from build123d import *

# Parameters (mm, degrees)
F0_R     = 30
F1_DEPTH = 3
F2_SIZE  = 2.99999
F3_R     = 19.125
F4_DEPTH = 3.001
F5_R     = 24.75
F5_R_2   = 22.75
F6_DEPTH = 20


# Not quite as in the source:
# - a fillet or chamfer is up to 0.001 mm smaller than in the source, because OpenCascade refuses the exact size


with BuildPart() as f1:
    # F0 (on Top) → F1 (new body)
    with BuildSketch(Plane.XY):
        Circle(F0_R)
    extrude(amount=F1_DEPTH)

    # F2 (size 3 in the source; OpenCascade refuses exactly that, so slightly less here)
    f2_edges = [f1.edges().sort_by_distance(p)[0] for p in [
        (-30, 0, 3),
    ]]
    chamfer(f2_edges, length=F2_SIZE)

    # F3 (on face) → F4 (cut, through all)
    with BuildSketch(Plane.XY.offset(3)):
        Circle(F3_R)
    extrude(amount=-F4_DEPTH, mode=Mode.SUBTRACT)

    # F5 (on face) → F6 (join)
    with BuildSketch(Plane(origin=(0, 0, 0), x_dir=(1, 0, 0), z_dir=(0, 0, -1))):
        Circle(F5_R)
        Circle(F5_R_2, mode=Mode.SUBTRACT)
    extrude(amount=F6_DEPTH)


solid = f1.part
Here's how the part is built. I have some questions about the finished solid (model axes, mm). A direction names the side the tool comes from. Give positions to 0.01 mm unless a question says otherwise; leave off trailing zeros. Write each loop counter-clockwise with the first axis right and the second up, starting at its lowest first coordinate (ties: lowest second). Pieces come first, ordered by that corner, then holes. Notation, with made-up numbers: (20.5, 20) -> (46.5, 20) arc R15 cw to (46.5, 35) -> close; hole circle Ø5 at (66, -30). An arc over 180 degrees is marked (long way). Use one line per item in the form item = value. Start each with the question number.
1. Thinking about a two-plate mould opening in Y: for faces 1 (the face through (-6.4, 18.4, 3)), 2 (the face through (-3.534, 26.915, 2.854)), 3 (the face through (-15.177, -11.637, 1.521)), 4 (the face through (-5, 19, 0)), which applies, +Y half, -Y half, draft (parallel to the pull), parting line (faces both ways), or undercut?
2. Will these pins go through, and if not, where does the flat tip stop? pin 1 Ø10 at (x, y) = (17, -4) entering from -Z; pin 2 Ø12 at (y, z) = (6, -14.5) entering from -X; pin 3 Ø12 at (x, z) = (11.5, -9) entering from -Y.
3. Imagine slicing it at D-D on z = 1. List the corners of the cut face in (x, y) for me (3 decimals), plus the area to 3 significant figures.
4. On a 3-axis mill with a long thin cutter (end or side, diameter ignored), from which of +Z, -Z, +X, -X, +Y, -Y can I reach the whole of each face in a straight line? I mean faces 5 (the face through (7, 22, -20)), 6 (the face through (4, 25, 0)). Say none if no direction works.
5. If I drill on L1, parallel to Y at x = 0, z = -15; L2, parallel to Z at x = -2.5, y = 20, over which ranges is the centre line in solid material (lowest first)?
6. Imagine slicing it at C-C on z = -7.75. List the corners of the cut face in (x, y) for me.
Entries:
q1.face_1 = draft
q1.face_2 = parting line
q1.face_3 = undercut
q1.face_4 = undercut
q2.pin_1 = 0
q2.pin_2 = -24.75
q2.pin_3 = -24.13
q3.outline = circle Ø58 at (0, 0); hole circle Ø38.25 at (0, 0)
q3.area = 1,490 mm²
q4.face_5 = -Z, +X, -X, +Y, -Y
q4.face_6 = -Z
q5.L1 = -24.75 to -22.75, 22.75 to 24.75
q5.L2 = 0 to 3
q6.outline = circle Ø49.5 at (0, 0); hole circle Ø45.5 at (0, 0)
